The drawing under review shows one solid part. Ordinate dimensions are in mm from its lowest x, y, z. A direction names the side the tool comes from. Coordinates: 2 decimals unless noted, no trailing zeros. Write each loop counter-clockwise with the first axis right and the second up, starting at its lowest first coordinate (ties: lowest second). Pieces come first, ordered by that corner, then holes.
Q1. Add section D-D, the plane z = 22. Give the boundary of the cut face in (x, y).
Q2. Add section C-C, the plane y = 18.25. Give the boundary of the cut face in (x, z).
Q3. Clearance check with flat-ended pins moving along their axes: pin 1 Ø5 at (y, z) = (25, 76) entering from -X; pin 2 Ø3 at (x, z) = (10.34, 54.86) entering from -Y; pin 3 Ø3 at (x, z) = (14, 50) entering from +Y; pin 4 Ø15 at (x, z) = (21.5, 37.5) entering from -Y. State where each tip first meets the part, or that it passes through.
Q4. To check wall thickness, follow probe 1 along X at (y, z) = (19.5, 6.16); probe 2 along X at (y, z) = (13, 25.5); probe 3 along Y at (x, z) = (74, 68.5). State the ranges of each line that lie inside material, in increasing order.
Q5. Add section A-A, the plane z = 6.16. Give the boundary of the cut face in (x, y).
Q6. The part is to be moulded in two halves that separate along Y. For the marked faces 1, 2 and 3, say which applies: +Y half, -Y half, draft (parallel to the pull), parting line (faces both ways), or undercut.
Q7. Machinability: for the marked faces 4, 5 and 6, which of the approach directions +Z, -Z, +X, -X, +Y, -Y give a long, thin tool a straight path to every point of the face, cutting with its end or side? Answer none if there is none.
Q8. Add section B-B, the plane x = 65. Give the boundary of the cut face in (y, z).
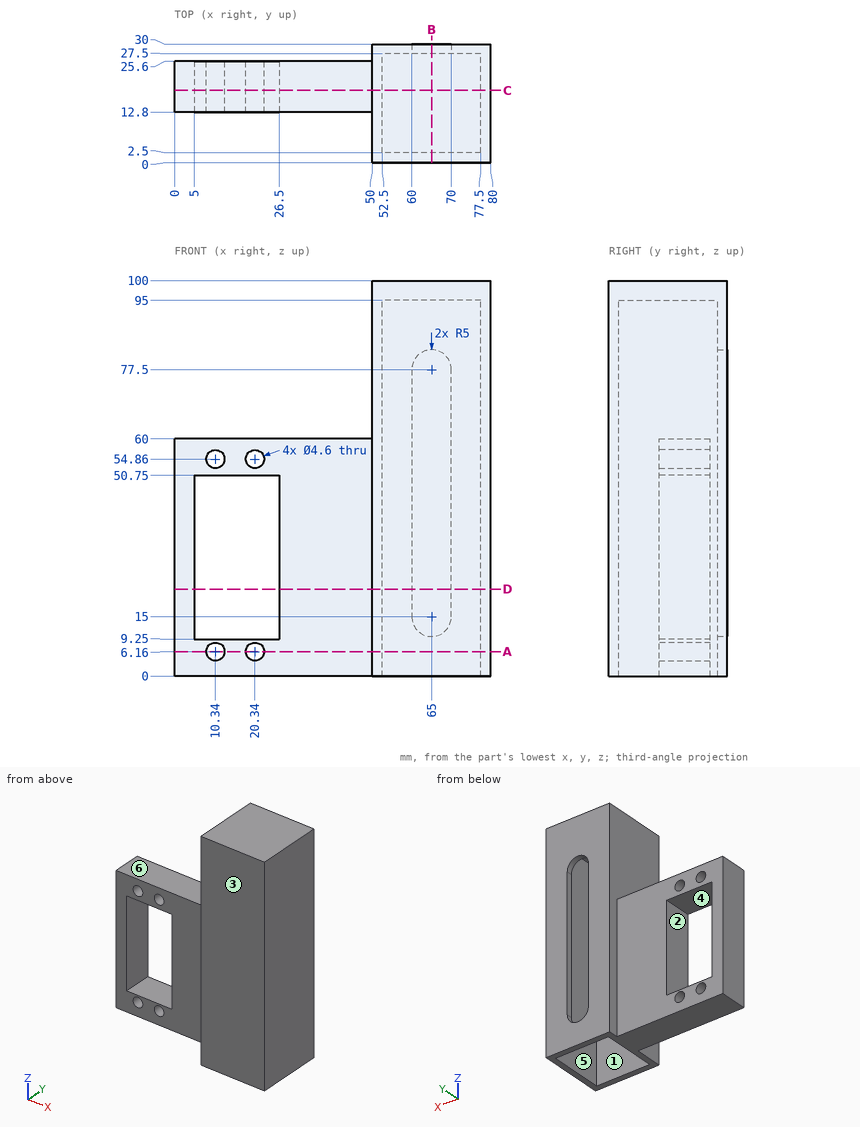
Here are the results:
1. outline: (0, 12.8) - (5, 12.8) - (5, 25.6) - (0, 25.6) - close; (26.5, 12.8) - (50, 12.8) - (50, 0) - (80, 0) - (80, 30) - (70, 30) - (70, 27.5) - (77.5, 27.5) - (77.5, 2.5) - (52.5, 2.5) - (52.5, 27.5) - (60, 27.5) - (60, 30) - (50, 30) - (50, 25.6) - (26.5, 25.6) - close
2. outline: (0, 0) - (52.5, 0) - (52.5, 95) - (77.5, 95) - (77.5, 0) - (80, 0) - (80, 100) - (50, 100) - (50, 60) - (0, 60) - close; hole (5, 9.25) - (26.5, 9.25) - (26.5, 50.75) - (5, 50.75) - close; hole circle Ø4.6 at (10.34, 6.16); hole circle Ø4.6 at (10.34, 54.86); hole circle Ø4.6 at (20.34, 6.16); hole circle Ø4.6 at (20.34, 54.86)
3. pin 1: stops at x = 50
3. pin 2: passes through
3. pin 3: stops at y = 25.6
3. pin 4: stops at y = 12.8
4. probe 1: x = 0 to 8.04, 12.64 to 18.04, 22.64 to 52.5, 77.5 to 80
4. probe 2: x = 0 to 5, 26.5 to 52.5, 77.5 to 80
4. probe 3: y = 0 to 2.5, 27.5 to 30
5. outline: (0, 12.8) - (8.04, 12.8) - (8.04, 25.6) - (0, 25.6) - close; (12.64, 12.8) - (18.04, 12.8) - (18.04, 25.6) - (12.64, 25.6) - close; (22.64, 12.8) - (50, 12.8) - (50, 0) - (80, 0) - (80, 30) - (50, 30) - (50, 25.6) - (22.64, 25.6) - close; hole (52.5, 2.5) - (77.5, 2.5) - (77.5, 27.5) - (52.5, 27.5) - close
6. face 1: undercut
6. face 2: draft
6. face 3: -Y half
7. face 4: +Y, -Y
7. face 5: -Z
7. face 6: +Z, -X, +Y, -Y
8. outline: (0, 0) - (2.5, 0) - (2.5, 95) - (27.5, 95) - (27.5, 82.5) - (30, 82.5) - (30, 100) - (0, 100) - close; (27.5, 0) - (30, 0) - (30, 10) - (27.5, 10) - close
